```python
from build123d import *

# Parameters (mm, degrees)
F0_W     = 150
F0_H     = 15
F0_R     = 3
F1_DEPTH = 4
F2_W     = 8
F2_H     = 15
F3_DEPTH = 25
F4_W     = 14.5
F4_H     = 7
F5_DEPTH = 200


with BuildPart() as f1:
    # F0 (on Front) → F1 (new body, symmetric)
    with BuildSketch(Plane.XZ):
        with Locations((67.5, 0)):
            Rectangle(F0_W, F0_H)
        Circle(F0_R, mode=Mode.SUBTRACT)
        with BuildLine():
            ThreePointArc((55, -3), (52, 0), (55, 3))
            Line((55, 3), (135, 3))
            ThreePointArc((135, 3), (138, 0), (135, -3))
            Line((135, -3), (55, -3))
        make_face(mode=Mode.SUBTRACT)
    extrude(amount=F1_DEPTH, both=True)

    # F2 (on face) → F3 (join)
    with BuildSketch(Plane.YZ.offset(142.5)):
        Rectangle(F2_W, F2_H)
    extrude(amount=F3_DEPTH)

    # F4 (on face) → F5 (join)
    with BuildSketch(Plane(origin=(0, 0, -7.5), x_dir=(1, 0, 0), z_dir=(0, 0, -1))):
        with Locations((155, 7.5)):
            Rectangle(F4_W, F4_H)
    extrude(amount=-F5_DEPTH)


solid = f1.part
```
Input: part model. Units: mm. Frame: model coordinates. A direction names the side the tool comes from. Coordinates: 2 decimals unless noted, no trailing zeros. Order: outer loops, then holes, each group sorted by start corner. A loop starts at its lowest first (then second) coordinate and runs counter-clockwise, first axis right, second up. Notation, with made-up numbers: (63, 28) - (82, 28) arc R32 ccw to (82, 63) - close; hole circle Ø5 at (82.5, -20.75). An arc over 180 degrees is marked (long way). Put each result on its own line as item: value.
1. Cut plane D-D on z = 43. Return the cut outline in (x, y).
Report:
outline: (147.75, -11) - (162.25, -11) - (162.25, -4) - (147.75, -4) - close
2. Draft query along Z for faces 4 (the face through (165, -4, 0)), 5 (the face through (79, 0, -7.5)), 6 (the face through (138, 0, 0)), 7 (the face through (79, 0, 7.5)). Return one class per face: pulls with the +Z half, pulls with the -Z half, needs draft (parallel to the pull), parting line crosses it, or undercut.
Report:
face 4: needs draft
face 5: pulls with the -Z half
face 6: undercut
face 7: pulls with the +Z half
3. Cut plane B-B on z = 0. Return the cut outline in (x, y), then the cut area to 4 significant figures.
Report:
outline: (-7.5, -4) - (-3, -4) - (-3, 4) - (-7.5, 4) - close; (3, -4) - (52, -4) - (52, 4) - (3, 4) - close; (138, -4) - (147.75, -4) - (147.75, -11) - (162.25, -11) - (162.25, -4) - (167.5, -4) - (167.5, 4) - (138, 4) - close
area: 765.5 mm2
4. Reachability of faces 1 (the face through (96, 0, -3)), 2 (the face through (155, -4, 99)), 3 (the face through (69, -4, -3.4)) from +Z, -Z, +X, -X, +Y, -Y: full face, straight path, thin tool, end or side. Return the list, or none.
Report:
face 1: +Y, -Y
face 2: +Z, +X, -X, +Y
face 3: +Z, -Z, -X, -Y
5. Line query: line 1 along Z through (x, y) = (0, 0.5); line 2 along X through (y, z) = (-8.5, 26); line 3 along Z through (x, y) = (144.5, 1.5). Output: solid intervals per line, ascending.
Report:
line 1: z = -7.5 to -3, 3 to 7.5
line 2: x = 147.75 to 162.25
line 3: z = -7.5 to 7.5
6. Cut plane C-C on y = 0.5. Return the cut outline in (x, z), then the cut area to 3 significant figures.
Report:
outline: (-7.5, -7.5) - (167.5, -7.5) - (167.5, 7.5) - (-7.5, 7.5) - close; hole circle Ø6 at (0, 0); hole (55, -3) - (135, -3) arc R3 ccw to (135, 3) - (55, 3) arc R3 ccw to start
area: 2,090 mm2
7. Cut plane A-A on x = 130. Return the cut outline in (y, z), then the cut area to 3 significant figures.
Report:
outline: (-4, -7.5) - (4, -7.5) - (4, -3) - (-4, -3) - close; (-4, 3) - (4, 3) - (4, 7.5) - (-4, 7.5) - close
area: 72.0 mm2
8. Contact query for flat-ended pins moving along their axis: pin 1 Ø6.5 at (x, y) = (54, 1) entering from +Z; pin 2 Ø8 at (x, z) = (0, 0) entering from +Y; pin 3 Ø3 at (y, z) = (-3, 139) entering from -X; pin 4 Ø12 at (x, z) = (108.5, 1.5) entering from -Y. Output: stop coordinate, or through.
Report:
pin 1: stops at z = 7.5
pin 2: stops at y = 4
pin 3: stops at x = 147.75
pin 4: stops at y = -4
